Work out the finished part from the listing and answer in its coordinate system (mm). Give positions to 0.01 mm unless a question says otherwise; leave off trailing zeros. Write each loop counter-clockwise with the first axis right and the second up, starting at its lowest first coordinate (ties: lowest second). Pieces come first, ordered by that corner, then holes. Notation, with made-up numbers: (84.25, 64) - (91.25, 64) arc R36 ccw to (91.25, 101) - close; hole circle Ø9 at (23.25, 18.25). An arc over 180 degrees is marked (long way). Write item = value, one per line.
from build123d import *

# Parameters (mm, degrees)
SKETCH1_W           = 70
SKETCH1_H           = 12
BOSS_EXTRUDE1_DEPTH = 3
SKETCH3_R           = 3
CUT_EXTRUDE1_DEPTH  = 36.637059362
SKETCH4_R           = 5
BOSS_EXTRUDE2_DEPTH = 8
FILLET2_R           = 0.5


with BuildPart() as part:
    # Sketch1 → Boss-Extrude1 (new body)
    with BuildSketch(Plane(origin=(0, 0, 0), x_dir=(1, 0, 0), z_dir=(0, 1, 0))):
        Rectangle(SKETCH1_W, SKETCH1_H)
    extrude(amount=BOSS_EXTRUDE1_DEPTH)

    # Sketch3 → Cut-Extrude1 (cut, through all)
    with BuildSketch(Plane(origin=(0, 3, 0), x_dir=(1, 0, 0), z_dir=(0, 1, 0))):
        with Locations(Location((-31, 0, 0), (0, 0, 270))):
            Circle(SKETCH3_R)
        with Locations(Location((31, 0, 0), (0, 0, 270))):
            Circle(SKETCH3_R)
    extrude(amount=-CUT_EXTRUDE1_DEPTH, mode=Mode.SUBTRACT)

    # Sketch4 → Boss-Extrude2 (add)
    with BuildSketch(Plane.XZ):
        with Locations(Location((0, 0, 0), (0, 0, 270))):
            Circle(SKETCH4_R)
    extrude(amount=BOSS_EXTRUDE2_DEPTH)

    # Fillet2
    fillet2_edges = [part.edges().sort_by_distance(p)[0] for p in [
        (0, 0, 5),
        (0, -8, 5),
    ]]
    fillet(fillet2_edges, radius=FILLET2_R)


solid = part.part
1. Find section C-C, the plane y = 1.5. Give the vertices of the cut face in (x, z), then the cut area to 3 significant figures.
Solution:
outline = (-35, -6) - (35, -6) - (35, 6) - (-35, 6) - close; hole circle Ø6 at (-31, 0); hole circle Ø6 at (31, 0)
area = 783 mm^2
2. Find section A-A, the plane x = -31. Give the vertices of the cut face in (y, z), then the cut area to 3 significant figures.
Solution:
outline = (0, -6) - (3, -6) - (3, -3) - (0, -3) - close; (0, 3) - (3, 3) - (3, 6) - (0, 6) - close
area = 18.0 mm^2
3. Find section D-D, the plane x = 0. Give the vertices of the cut face in (y, z).
Solution:
outline = (-8, -4.5) arc R0.5 ccw to (-7.5, -5) - (-0.5, -5) arc R0.5 cw to (0, -5.5) - (0, -6) - (3, -6) - (3, 6) - (0, 6) - (0, 5.5) arc R0.5 cw to (-0.5, 5) - (-7.5, 5) arc R0.5 ccw to (-8, 4.5) - close
4. Given pin 1 (3.5 mm diameter, centred on x = 15, z = -1.5, fed in from -Y); pin 2 (3 mm diameter, centred on y = -2, z = 2.5, fed in from +X); pin 3 (3 mm diameter, centred on y = -5, z = -2.5, fed in from -X), each flat-ended and moving along its own axis, determine where each tip first touches the part or whether it passes through.
Solution:
pin_1 = 0
pin_2 = 4.9
pin_3 = -4.9
5. For a pull along Z with two mould halves and no side action, classify faces 1 (the flat face through (0, 1, -6)), 2 (the cylindrical face through (-30.1, 1.52, 2.86)), 3 (the cylindrical face through (-4.88, -3.95, 1.08)) as pulls with the +Z half, pulls with the -Z half, needs draft (parallel to the pull), parting line crosses it, or undercut.
Solution:
face_1 = pulls with the -Z half
face_2 = undercut
face_3 = parting line crosses it
6. Find section B-B, the plane z = 0. Give the vertices of the cut face in (x, y).
Solution:
outline = (-35, 0) - (-34, 0) - (-34, 3) - (-35, 3) - close; (-28, 0) - (-5.5, 0) arc R0.5 cw to (-5, -0.5) - (-5, -7.5) arc R0.5 ccw to (-4.5, -8) - (4.5, -8) arc R0.5 ccw to (5, -7.5) - (5, -0.5) arc R0.5 cw to (5.5, 0) - (28, 0) - (28, 3) - (-28, 3) - close; (34, 0) - (35, 0) - (35, 3) - (34, 3) - close
7. Straight lines are drawn through the part: line 1 (X direction, y = 0.9, z = 0); line 2 (Y direction, x = -13, z = 1); line 3 (X direction, y = 1, z = 1). For each, find the intervals that lie inside material, in ascending order.
Solution:
line_1 = -35 to -34, -28 to 28, 34 to 35
line_2 = 0 to 3
line_3 = -35 to -33.83, -28.17 to 28.17, 33.83 to 35
